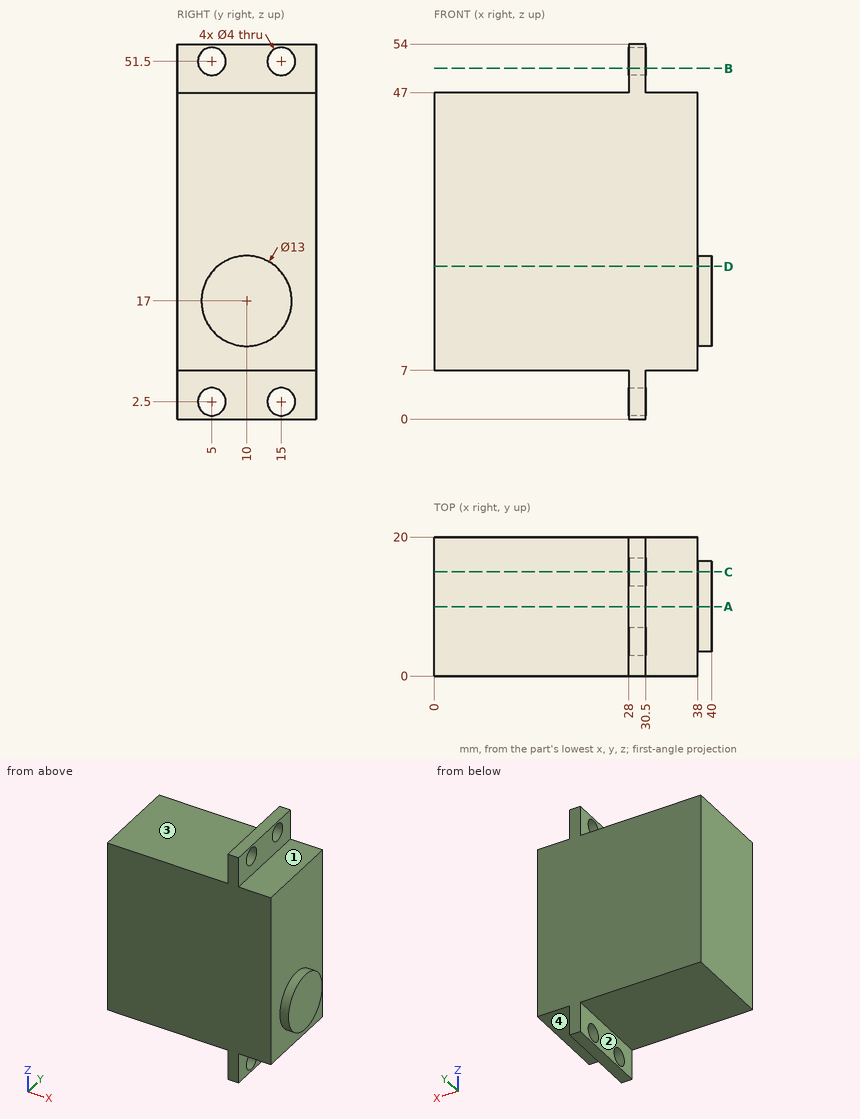
Here's the drawing with two shaded views (mm, measured from the low corner). I have some questions. A direction names the side the tool comes from. Coordinates: 2 decimals unless noted, no trailing zeros. Loops run counter-clockwise (first coordinate to the right, second up) from the corner with the lowest first, then second, coordinate; pieces in that order, holes last. Notation, with made-up numbers: (-4.75, 74) - (2.25, 74) arc R24 ccw to (2.25, 90) - close; hole circle Ø3 at (-5, 63.5). An arc over 180 degrees is marked (long way). Answer as CSV lines item,"result". Start each with the question number.
1) Suppose I cut it at B-B (z = 50.5). Please give me the cut outline in (x, y), plus the area to 3 significant figures.
2) Suppose I cut it at A-A (y = 10). Please give me the cut outline in (x, z), plus the area to 3 significant figures.
3) Which directions (+Z, -Z, +X, -X, +Y, -Y) give clear straight access to the entire face, cutting with the end or side of a thin tool? Please do the marked faces 1, 2, 3 and 4.
4) Suppose I cut it at C-C (y = 15). Please give me the cut outline in (x, z), plus the area to 3 significant figures.
5) Suppose I cut it at D-D (z = 22). Please give me the cut outline in (x, y), plus the area to 3 significant figures.
6) For pin 1 (6 mm diameter, centred on x = 17, y = 8, fed in from +Z); pin 2 (4.5 mm diameter, centred on y = 5, z = 51.5, fed in from +X); pin 3 (5.5 mm diameter, centred on y = 14.5, z = 49.5, fed in from +X), each with a flat end and sliding along its axis, tell me the tip position at first contact or that it passes through.
7) I need wall thicknesses on line 1 (Y direction, x = 30.05, z = 2.5); line 2 (Y direction, x = 29, z = 51); line 3 (X direction, y = 7.5, z = 46). Which ranges of each line are inside material? Lowest first, please. Write a range as from..to.
Check result:
1,outline,"(28, 0) - (30.5, 0) - (30.5, 3.27) - (28, 3.27) - close; (28, 6.73) - (30.5, 6.73) - (30.5, 13.27) - (28, 13.27) - close; (28, 16.73) - (30.5, 16.73) - (30.5, 20) - (28, 20) - close"
1,area,"32.7 mm²"
2,outline,"(0, 7) - (28, 7) - (28, 0) - (30.5, 0) - (30.5, 7) - (38, 7) - (38, 10.5) - (40, 10.5) - (40, 23.5) - (38, 23.5) - (38, 47) - (30.5, 47) - (30.5, 54) - (28, 54) - (28, 47) - (0, 47) - close"
2,area,"1,580 mm²"
3,face 1,"+Z, +X, +Y, -Y"
3,face 2,"-Z, -X, +Y, -Y"
3,face 3,"+Z, -X, +Y, -Y"
3,face 4,"-Z, +X, +Y, -Y"
4,outline,"(0, 7) - (28, 7) - (28, 4.5) - (30.5, 4.5) - (30.5, 7) - (38, 7) - (38, 12.85) - (40, 12.85) - (40, 21.15) - (38, 21.15) - (38, 47) - (30.5, 47) - (30.5, 49.5) - (28, 49.5) - (28, 47) - (0, 47) - close; (28, 0) - (30.5, 0) - (30.5, 0.5) - (28, 0.5) - close; (28, 53.5) - (30.5, 53.5) - (30.5, 54) - (28, 54) - close"
4,area,"1,550 mm²"
5,outline,"(0, 0) - (38, 0) - (38, 5.85) - (40, 5.85) - (40, 14.15) - (38, 14.15) - (38, 20) - (0, 20) - close"
5,area,"777 mm²"
6,pin 1,"stops at z = 47"
6,pin 2,"stops at x = 30.5"
6,pin 3,"stops at x = 38"
7,line 1,"y = 0..3, 7..13, 17..20"
7,line 2,"y = 0..3.06, 6.94..13.06, 16.94..20"
7,line 3,"x = 0..38"
